Here's how the part is built. I have some questions about the finished solid (model axes, mm). A direction names the side the tool comes from. Coordinates: 2 decimals unless noted, no trailing zeros. Order: outer loops, then holes, each group sorted by start corner. A loop starts at its lowest first (then second) coordinate and runs counter-clockwise, first axis right, second up. Notation, with made-up numbers: (-23.5, 49.25) - (16.5, 49.25) arc R27 ccw to (16.5, 76.25) - close; hole circle Ø4 at (87.25, -37.5). An arc over 180 degrees is marked (long way). Answer as CSV lines item,"result". Start each with the question number.
Item 1: Imagine slicing it at B-B on z = -4. List the corners of the cut face in (x, y) for me.
Item 2: I'm going to push flat-ended pins straight in: pin 1 (3.5 mm diameter, centred on y = -1, z = -2.5, fed in from +X); pin 2 (5.5 mm diameter, centred on x = 14.5, y = -15.5, fed in from -Z); pin 3 (1.4 mm diameter, centred on y = 14.5, z = -13, fed in from -X). Where does each tip first touch, or does it pass through?
Item 3: On a 3-axis mill with a long thin cutter (end or side, diameter ignored), from which of +Z, -Z, +X, -X, +Y, -Y can I reach the whole of each face in a straight line? I mean faces 4 (the face through (-10.5, 15, -13)), 5 (the face through (0, -17, -12.5)), 6 (the face through (5, 0, 7)), 7 (the face through (-15, -10.5, -13)), 8 (the face through (15, 10.5, -13)). Say none if no direction works.
Item 4: I need wall thicknesses on line 1 (Y direction, x = -12.7, z = 4.1); line 2 (X direction, y = -12, z = 4). Which ranges of each line are inside material? Lowest first, please.
Item 5: Imagine slicing it at A-A on z = 6. List the corners of the cut face in (x, y) for me.
Item 6: We'd pull the mould along X, two halves only. Please class faces 1 (the face through (0, -17, -7)), 2 (the face through (-14, -14, -12)), 3 (the face through (17.5, 0, -9)): pulls with the +X half, pulls with the -X half, needs draft (parallel to the pull), parting line crosses it, or undercut.
from build123d import *

# Parameters (mm, degrees)
F0_W      = 35
F0_H      = 35
F1_DEPTH  = 5
F2_R      = 11
F2_R_2    = 4
F3_DEPTH  = 2
F4_SIZE   = 2
F5_R      = 2.5
F6_DEPTH  = 13
F8_D      = 3.3
F8_DEPTH  = 3
F8_TIP    = 0.9914200214
F9_SIZE   = 0.5
F11_DEPTH = 7
F13_DEPTH = 2
F14_W     = 35
F14_H     = 35
F15_DEPTH = 7
F16_SIZE  = 2
F18_DEPTH = 2
F19_W     = 8
F19_H     = 5.5
F20_DEPTH = 1
F22_DEPTH = 2
F23_SIZE  = 0.2


with BuildPart() as f1:
    # F0 (on Top) → F1 (new body)
    with BuildSketch(Plane.XY):
        Rectangle(F0_W, F0_H)
    extrude(amount=F1_DEPTH)

    # F2 (on face) → F3 (join)
    with BuildSketch(Plane.XY.offset(5)):
        Circle(F2_R)
        Circle(F2_R_2, mode=Mode.SUBTRACT)
    extrude(amount=F3_DEPTH)

    # F4
    f4_edges = [f1.edges().sort_by_distance(p)[0] for p in [
        (-17.5, 17.5, 2.5),
        (-17.5, -17.5, 2.5),
        (17.5, -17.5, 2.5),
        (17.5, 17.5, 2.5),
    ]]
    chamfer(f4_edges, length=F4_SIZE)

    # F5 (on face) → F6 (join)
    with BuildSketch(Plane.XY.offset(5)):
        Circle(F5_R)
    extrude(amount=F6_DEPTH)

    # F8
    with Locations(Plane.XY.offset(5)):
        with Locations((-12.7, -12.7), (-12.7, 12.7), (12.7, 12.7), (12.7, -12.7)):
            Hole(F8_D / 2, depth=F8_DEPTH)
            with Locations((0, 0, -(F8_DEPTH + F8_TIP / 2))):  # 118° drill point
                Cone(0, F8_D / 2, F8_TIP, mode=Mode.SUBTRACT)

    # F9
    f9_edges = [f1.edges().sort_by_distance(p)[0] for p in [
        (0, -17.5, 5),
        (-17.5, 0, 5),
        (0, 17.5, 5),
        (17.5, 0, 5),
        (16.5, -16.5, 5),
        (16.5, 16.5, 5),
        (-16.5, 16.5, 5),
        (-16.5, -16.5, 5),
        (-11, 0, 7),
        (-4, 0, 7),
        (-2.5, 0, 18),
    ]]
    chamfer(f9_edges, length=F9_SIZE)

    # F10 (on face) → F11 (join)
    with BuildSketch(Plane(origin=(0, 0, 0), x_dir=(1, 0, 0), z_dir=(0, 0, -1))):
        with BuildLine():
            Line((10.4, 17.4), (-10.4, 17.4))
            ThreePointArc((-10.4, 17.4), (-15.3497474683, 15.3497474683), (-17.4, 10.4))
            Line((-17.4, 10.4), (-17.4, -10.4))
            ThreePointArc((-17.4, -10.4), (-15.3497474683, -15.3497474683), (-10.4, -17.4))
            Line((-10.4, -17.4), (10.4, -17.4))
            ThreePointArc((10.4, -17.4), (15.3497474683, -15.3497474683), (17.4, -10.4))
            Line((17.4, -10.4), (17.4, 10.4))
            ThreePointArc((17.4, 10.4), (15.3497474683, 15.3497474683), (10.4, 17.4))
        make_face()
    extrude(amount=F11_DEPTH)

    # F12 (on face) → F13 (join)
    with BuildSketch(Plane(origin=(0, 0, 0), x_dir=(1, 0, 0), z_dir=(0, 0, -1))):
        with BuildLine():
            Line((-10.5, 17.5), (-15.5, 17.5))
            Line((-15.5, 17.5), (-17.5, 15.5))
            Line((-17.5, 15.5), (-17.5, 10.5))
            Line((-17.5, 10.5), (-17.3992856778, 10.5))
            ThreePointArc((-17.3992856778, 10.5), (-15.3497474683, 15.3497474683), (-10.5, 17.3992856778))
            Line((-10.5, 17.3992856778), (-10.5, 17.5))
        make_face()
        with BuildLine():
            Line((15.5, 17.5), (10.5, 17.5))
            Line((10.5, 17.5), (10.5, 17.3992856778))
            ThreePointArc((10.5, 17.3992856778), (15.3497474683, 15.3497474683), (17.3992856778, 10.5))
            Line((17.3992856778, 10.5), (17.5, 10.5))
            Line((17.5, 10.5), (17.5, 15.5))
            Line((17.5, 15.5), (15.5, 17.5))
        make_face()
        with BuildLine():
            Line((17.5, -15.5), (17.5, -10.5))
            Line((17.5, -10.5), (17.3992856778, -10.5))
            ThreePointArc((17.3992856778, -10.5), (15.3497474683, -15.3497474683), (10.5, -17.3992856778))
            Line((10.5, -17.3992856778), (10.5, -17.5))
            Line((10.5, -17.5), (15.5, -17.5))
            Line((15.5, -17.5), (17.5, -15.5))
        make_face()
        with BuildLine():
            Line((-17.3992856778, -10.5), (-17.5, -10.5))
            Line((-17.5, -10.5), (-17.5, -15.5))
            Line((-17.5, -15.5), (-15.5, -17.5))
            Line((-15.5, -17.5), (-10.5, -17.5))
            Line((-10.5, -17.5), (-10.5, -17.3992856778))
            ThreePointArc((-10.5, -17.3992856778), (-15.3497474683, -15.3497474683), (-17.3992856778, -10.5))
        make_face()
    extrude(amount=F13_DEPTH)

    # F14 (on face) → F15 (join)
    with BuildSketch(Plane(origin=(0, 0, -7), x_dir=(1, 0, 0), z_dir=(0, 0, -1))):
        Rectangle(F14_W, F14_H)
        with BuildLine():
            Line((-10.4, 17.4), (10.4, 17.4))
            ThreePointArc((10.4, 17.4), (15.3497474683, 15.3497474683), (17.4, 10.4))
            Line((17.4, 10.4), (17.4, -10.4))
            ThreePointArc((17.4, -10.4), (15.3497474683, -15.3497474683), (10.4, -17.4))
            Line((10.4, -17.4), (-10.4, -17.4))
            ThreePointArc((-10.4, -17.4), (-15.3497474683, -15.3497474683), (-17.4, -10.4))
            Line((-17.4, -10.4), (-17.4, 10.4))
            ThreePointArc((-17.4, 10.4), (-15.3497474683, 15.3497474683), (-10.4, 17.4))
        make_face(mode=Mode.SUBTRACT)
        with BuildLine():
            ThreePointArc((17.4, 10.4), (15.3497474683, 15.3497474683), (10.4, 17.4))
            Line((10.4, 17.4), (-10.4, 17.4))
            ThreePointArc((-10.4, 17.4), (-15.3497474683, 15.3497474683), (-17.4, 10.4))
            Line((-17.4, 10.4), (-17.4, -10.4))
            ThreePointArc((-17.4, -10.4), (-15.3497474683, -15.3497474683), (-10.4, -17.4))
            Line((-10.4, -17.4), (10.4, -17.4))
            ThreePointArc((10.4, -17.4), (15.3497474683, -15.3497474683), (17.4, -10.4))
            Line((17.4, -10.4), (17.4, 10.4))
        make_face()
    extrude(amount=F15_DEPTH)

    # F16
    f16_edges = [f1.edges().sort_by_distance(p)[0] for p in [
        (-17.5, -17.5, -10.5),
        (17.5, -17.5, -10.5),
        (17.5, 17.5, -10.5),
        (-17.5, 17.5, -10.5),
    ]]
    chamfer(f16_edges, length=F16_SIZE)

    # F17 (on face) → F18 (join)
    with BuildSketch(Plane.XY.offset(-7)):
        with BuildLine():
            Line((15.5, 17.5), (10.5, 17.5))
            Line((10.5, 17.5), (10.5, 17.3992856778))
            ThreePointArc((10.5, 17.3992856778), (15.3497474683, 15.3497474683), (17.3992856778, 10.5))
            Line((17.3992856778, 10.5), (17.5, 10.5))
            Line((17.5, 10.5), (17.5, 15.5))
            Line((17.5, 15.5), (15.5, 17.5))
        make_face()
        with BuildLine():
            Line((-10.5, 17.5), (-15.5, 17.5))
            Line((-15.5, 17.5), (-17.5, 15.5))
            Line((-17.5, 15.5), (-17.5, 10.5))
            Line((-17.5, 10.5), (-17.3992856778, 10.5))
            ThreePointArc((-17.3992856778, 10.5), (-15.3497474683, 15.3497474683), (-10.5, 17.3992856778))
            Line((-10.5, 17.3992856778), (-10.5, 17.5))
        make_face()
        with BuildLine():
            Line((-17.3992856778, -10.5), (-17.5, -10.5))
            Line((-17.5, -10.5), (-17.5, -15.5))
            Line((-17.5, -15.5), (-15.5, -17.5))
            Line((-15.5, -17.5), (-10.5, -17.5))
            Line((-10.5, -17.5), (-10.5, -17.3992856778))
            ThreePointArc((-10.5, -17.3992856778), (-15.3497474683, -15.3497474683), (-17.3992856778, -10.5))
        make_face()
        with BuildLine():
            Line((17.5, -15.5), (17.5, -10.5))
            Line((17.5, -10.5), (17.3992856778, -10.5))
            ThreePointArc((17.3992856778, -10.5), (15.3497474683, -15.3497474683), (10.5, -17.3992856778))
            Line((10.5, -17.3992856778), (10.5, -17.5))
            Line((10.5, -17.5), (15.5, -17.5))
            Line((15.5, -17.5), (17.5, -15.5))
        make_face()
    extrude(amount=F18_DEPTH)

    # F19 (on face) → F20 (cut)
    with BuildSketch(Plane.XZ.offset(17.5)):
        with Locations((0, -9.75)):
            Rectangle(F19_W, F19_H)
    extrude(amount=-F20_DEPTH, mode=Mode.SUBTRACT)

    # F21 (on face) → F22 (cut)
    with BuildSketch(Plane(origin=(0, 0, -14), x_dir=(1, 0, 0), z_dir=(0, 0, -1))):
        with BuildLine():
            Line((-17.5, 15.5), (-17.5, 10.5))
            Line((-17.5, 10.5), (-12.5, 10.5))
            ThreePointArc((-12.5, 10.5), (-11.0857864376, 11.0857864376), (-10.5, 12.5))
            Line((-10.5, 12.5), (-10.5, 17.5))
            Line((-10.5, 17.5), (-15.5, 17.5))
            Line((-15.5, 17.5), (-17.5, 15.5))
        make_face()
        with BuildLine():
            Line((15.5, 17.5), (10.5, 17.5))
            Line((10.5, 17.5), (10.5, 12.5))
            ThreePointArc((10.5, 12.5), (11.0857864376, 11.0857864376), (12.5, 10.5))
            Line((12.5, 10.5), (17.5, 10.5))
            Line((17.5, 10.5), (17.5, 15.5))
            Line((17.5, 15.5), (15.5, 17.5))
        make_face()
        with BuildLine():
            Line((10.5, -12.5), (10.5, -17.5))
            Line((10.5, -17.5), (15.5, -17.5))
            Line((15.5, -17.5), (17.5, -15.5))
            Line((17.5, -15.5), (17.5, -10.5))
            Line((17.5, -10.5), (12.5, -10.5))
            ThreePointArc((12.5, -10.5), (11.0857864376, -11.0857864376), (10.5, -12.5))
        make_face()
        with BuildLine():
            Line((-12.5, -10.5), (-17.5, -10.5))
            Line((-17.5, -10.5), (-17.5, -15.5))
            Line((-17.5, -15.5), (-15.5, -17.5))
            Line((-15.5, -17.5), (-10.5, -17.5))
            Line((-10.5, -17.5), (-10.5, -12.5))
            ThreePointArc((-10.5, -12.5), (-11.0857864376, -11.0857864376), (-12.5, -10.5))
        make_face()
    extrude(amount=-F22_DEPTH, mode=Mode.SUBTRACT)

    # F23
    f23_edges = [f1.edges().sort_by_distance(p)[0] for p in [
        (17.5, 0, -14),
        (0, -17.5, -14),
        (-17.5, 0, -14),
        (0, 17.5, -14),
        (10.5, 15, -14),
        (11.085786, 11.085786, -14),
        (15, 10.5, -14),
        (15, -10.5, -14),
        (11.085786, -11.085786, -14),
        (10.5, -15, -14),
        (-10.5, -15, -14),
        (-11.085786, -11.085786, -14),
        (-15, -10.5, -14),
        (-15, 10.5, -14),
        (-11.085786, 11.085786, -14),
        (-10.5, 15, -14),
    ]]
    chamfer(f23_edges, length=F23_SIZE)


solid = f1.part
Responses:
1,outline,"(-17.4, -10.4) arc R7 ccw to (-10.4, -17.4) - (10.4, -17.4) arc R7 ccw to (17.4, -10.4) - (17.4, 10.4) arc R7 ccw to (10.4, 17.4) - (-10.4, 17.4) arc R7 ccw to (-17.4, 10.4) - close"
2,pin 1,"stops at x = 17.4"
2,pin 2,"stops at z = -12"
2,pin 3,"stops at x = -10.5"
3,face 4,"-Z, -X, +Y"
3,face 5,"-Y"
3,face 6,"+Z"
3,face 7,"-Z, -X, -Y"
3,face 8,"-Z, +X, +Y"
4,line 1,"y = -17.5 to -14.35, -11.05 to 11.05, 14.35 to 17.5"
4,line 2,"x = -17.5 to -14.19, -11.21 to 11.21, 14.19 to 17.5"
5,outline,"circle Ø22 at (0, 0); circle Ø5 at (0, 0); hole circle Ø8 at (0, 0)"
6,face 1,"undercut"
6,face 2,"needs draft"
6,face 3,"pulls with the +X half"
